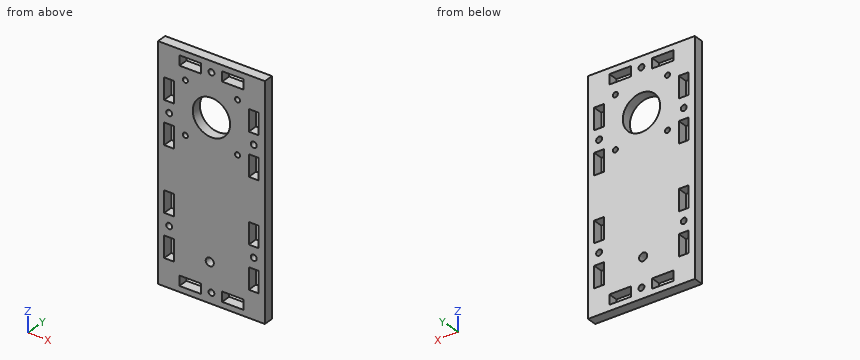
```python
from build123d import *

# Parameters (mm, degrees)
F0_W     = 63.5
F0_H     = 136.525
F0_W_2   = 12.7
F0_H_2   = 5.842
F0_R     = 2.413
F0_R_2   = 1.7526
F0_R_3   = 1.5
F0_R_4   = 11.1125
F1_DEPTH = 5.842
F2_W     = 5.842
F2_H     = 12.7
F2_R     = 1.7526
F3_DEPTH = 25.4


with BuildPart() as f1:
    # F0 (on Front) → F1 (new body)
    with BuildSketch(Plane.XZ):
        Rectangle(F0_W, F0_H)
        with Locations((-12.7, -61.9125)):
            Rectangle(F0_W_2, F0_H_2, mode=Mode.SUBTRACT)
        with Locations((-1, -44.9875)):
            Circle(F0_R, mode=Mode.SUBTRACT)
        with Locations((0, -61.9125)):
            Circle(F0_R_2, mode=Mode.SUBTRACT)
        with Locations((12.7, -61.9125)):
            Rectangle(F0_W_2, F0_H_2, mode=Mode.SUBTRACT)
        with Locations((-15.5, 21.0125)):
            Circle(F0_R_3, mode=Mode.SUBTRACT)
        with Locations((-15.5, 52.0125)):
            Circle(F0_R_3, mode=Mode.SUBTRACT)
        with Locations((-12.7, 61.9125)):
            Rectangle(F0_W_2, F0_H_2, mode=Mode.SUBTRACT)
        with Locations((15.5, 21.0125)):
            Circle(F0_R_3, mode=Mode.SUBTRACT)
        with Locations((0, 36.5125)):
            Circle(F0_R_4, mode=Mode.SUBTRACT)
        with Locations((0, 61.9125)):
            Circle(F0_R_2, mode=Mode.SUBTRACT)
        with Locations((15.5, 52.0125)):
            Circle(F0_R_3, mode=Mode.SUBTRACT)
        with Locations((12.7, 61.9125)):
            Rectangle(F0_W_2, F0_H_2, mode=Mode.SUBTRACT)
    extrude(amount=F1_DEPTH)

    # F2 (on face) → F3 (cut)
    with BuildSketch(Plane.XZ.offset(5.842)):
        with Locations((-25.146, 42.8625)):
            Rectangle(F2_W, F2_H)
        with Locations((-25.146, 17.4625)):
            Rectangle(F2_W, F2_H)
        with Locations((-25.146, 30.1625)):
            Circle(F2_R)
        with Locations((25.146, 17.4625)):
            Rectangle(F2_W, F2_H)
        with Locations((25.146, 42.8625)):
            Rectangle(F2_W, F2_H)
        with Locations((25.146, 30.1625)):
            Circle(F2_R)
        with Locations((-25.146, -20.6375)):
            Rectangle(F2_W, F2_H)
        with Locations((-25.146, -33.3375)):
            Circle(F2_R)
        with Locations((-25.146, -46.0375)):
            Rectangle(F2_W, F2_H)
        with Locations((25.146, -20.6375)):
            Rectangle(F2_W, F2_H)
        with Locations((25.146, -46.0375)):
            Rectangle(F2_W, F2_H)
        with Locations((25.146, -33.3375)):
            Circle(F2_R)
    extrude(amount=-F3_DEPTH, mode=Mode.SUBTRACT)


solid = f1.part
```
Can you work these out from the model? Positions are in its coordinate system, mm. Coordinates: 2 decimals unless noted, no trailing zeros. Loops run counter-clockwise (first coordinate to the right, second up) from the corner with the lowest first, then second, coordinate; pieces in that order, holes last.
Item 1: Suppose I cut it at C-C (x = 4). Please give me the cut outline in (y, z), then the cut area to 3 significant figures.
Answers below:
outline: (-5.84, -68.26) - (0, -68.26) - (0, 26.14) - (-5.84, 26.14) - close; (-5.84, 46.88) - (0, 46.88) - (0, 68.26) - (-5.84, 68.26) - close
area: 676 mm2
Item 2: Please list where these lines run through material, in increasing order: L1, parallel to X at y = -3.45, z = 60; L2, parallel to Z at x = 27.5, y = -3.75; L3, parallel to Z at x = 17.5, y = -4.1.
Answers below:
L1: x = -31.75 to -19.05, -6.35 to 6.35, 19.05 to 31.75
L2: z = -68.26 to -52.39, -39.69 to -26.99, -14.29 to 11.11, 23.81 to 36.51, 49.21 to 68.26
L3: z = -68.26 to -64.83, -58.99 to 58.99, 64.83 to 68.26
Item 3: Suppose I cut it at D-D (y = -3.3). State how many separate pieces and enclosed holes the cut face has, then the cut area to 3 significant figures.
Answers below:
separate pieces: 1
enclosed holes: 24
area: 7,290 mm2
Item 4: Suppose I cut it at A-A (x = 15.5). Please give me the cut outline in (y, z).
Answers below:
outline: (-5.84, -68.26) - (0, -68.26) - (0, -64.83) - (-5.84, -64.83) - close; (-5.84, -58.99) - (0, -58.99) - (0, 19.51) - (-5.84, 19.51) - close; (-5.84, 22.51) - (0, 22.51) - (0, 50.51) - (-5.84, 50.51) - close; (-5.84, 53.51) - (0, 53.51) - (0, 58.99) - (-5.84, 58.99) - close; (-5.84, 64.83) - (0, 64.83) - (0, 68.26) - (-5.84, 68.26) - close
Item 5: Suppose I cut it at B-B (z = -25). Please give me the cut outline in (x, y) (3 decimals).
Answers below:
outline: (-31.75, -5.842) - (-28.067, -5.842) - (-28.067, 0) - (-31.75, 0) - close; (-22.225, -5.842) - (22.225, -5.842) - (22.225, 0) - (-22.225, 0) - close; (28.067, -5.842) - (31.75, -5.842) - (31.75, 0) - (28.067, 0) - close
